Design review of the part built by this model. Coordinates are the model's own, in mm. Face numbers are marked on the shaded views. A direction names the side the tool comes from. Give positions to 0.01 mm unless a question says otherwise; leave off trailing zeros. Write each loop counter-clockwise with the first axis right and the second up, starting at its lowest first coordinate (ties: lowest second). Pieces come first, ordered by that corner, then holes. Notation, with made-up numbers: (35, 72.5) - (81, 72.5) arc R12 ccw to (81, 76.5) - close; hole circle Ø2 at (-1, -24.75). An arc over 180 degrees is marked (long way). Write each question's results on one line, items separated by ' | '. Start each with the question number.
from build123d import *

# Parameters (mm, degrees)
F0_W     = 23
F0_H     = 35
F1_DEPTH = 4.25
F2_W     = 3.5
F2_H     = 35
F3_DEPTH = 17
F4_W     = 6.35
F4_H     = 25
F5_DEPTH = 4.251
F6_R     = 1.15
F7_DEPTH = 3.501


with BuildPart() as f1:
    # F0 (on Front) → F1 (new body)
    with BuildSketch(Plane.XZ):
        with Locations((0.065487, 0)):
            Rectangle(F0_W, F0_H)
    extrude(amount=-F1_DEPTH)

    # F2 (on face) → F3 (join)
    with BuildSketch(Plane.XZ):
        with Locations((-9.684513, 0)):
            Rectangle(F2_W, F2_H)
    extrude(amount=F3_DEPTH)

    # F4 (on face) → F5 (cut, through all)
    with BuildSketch(Plane.XZ):
        with Locations((1.815487, 0)):
            Rectangle(F4_W, F4_H)
    extrude(amount=-F5_DEPTH, mode=Mode.SUBTRACT)

    # F6 (on face) → F7 (cut, through all)
    with BuildSketch(Plane.YZ.offset(-7.934513)):
        with Locations((-13, 12.5)):
            Circle(F6_R)
        with Locations((-6, 12.5)):
            Circle(F6_R)
    extrude(amount=-F7_DEPTH, mode=Mode.SUBTRACT)


solid = f1.part
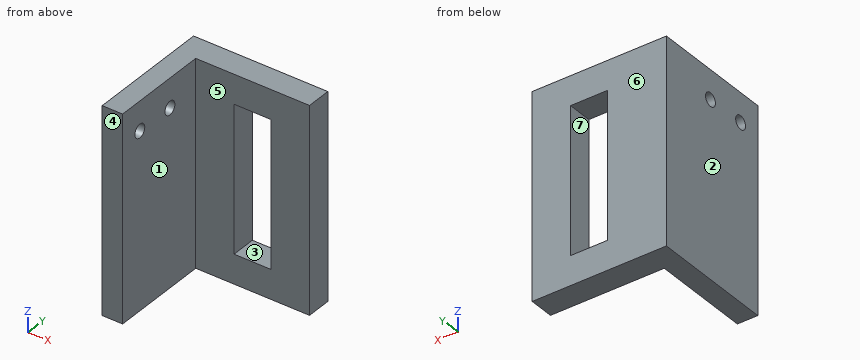
Q1. Add section A-A on z = 8. State the section outline as (x, y) points.
Q2. Add section C-C on y = -6. State the section outline as (x, z) points, plus the area to 3 significant figures.
Q3. Machinability: for the marked faces 5, 6 and 7, which of the approach directions +Z, -Z, +X, -X, +Y, -Y give a long, thin tool a straight path to every point of the face, cutting with its end or side? Answer none if there is none.
Q4. For line 1 along Z through (x, y) = (2.25, 2.25); line 2 along Z through (x, y) = (-9.3, -6); line 3 along X through (y, z) = (1, -0.5), list the stretches that pass through material, from the lowest coordinate up. Write a range as [from, to].
Q5. Add section B-B on x = 4.5. State the section outline as (y, z) points.
Q6. Insertion check: P1, Ø5, axis at y = -3.5, z = -12, coming from the +X side; P2, Ø6, axis at x = 5.5, z = -2.5, coming from the -Y side; P3, Ø1.8, axis at y = -13, z = 12.5, coming from the +X side. Each pin has a flat end and moves straight along its axis. Give the tip position at first contact, or say it passes through.
Q7. Add section D-D on z = -14. State the section outline as (x, y) points.
Q8. The part is to be moulded in two halves that separate along X. For the marked faces 1, 2, 3 and 4, say which applies: +X half, -X half, draft (parallel to the pull), parting line (faces both ways), or undercut.
Result:
1) outline: (-11.43, -17) - (-7.93, -17) - (-7.93, 0) - (-1.36, 0) - (-1.36, 4.25) - (-11.43, 4.25) - close; (4.99, 0) - (11.57, 0) - (11.57, 4.25) - (4.99, 4.25) - close
2) outline: (-11.43, -17.5) - (-7.93, -17.5) - (-7.93, 11.35) - (-11.43, 11.35) - close; (-11.43, 13.65) - (-7.93, 13.65) - (-7.93, 17.5) - (-11.43, 17.5) - close | area: 114 mm²
3) face 5: +Z, -Z, +X, -Y | face 6: +Z, -Z, +X, -X, +Y | face 7: +Y, -Y
4) line 1: z = [-17.5, -12.5], [12.5, 17.5] | line 2: z = [-17.5, 11.35], [13.65, 17.5] | line 3: x = [-11.43, -1.36], [4.99, 11.57]
5) outline: (0, -17.5) - (4.25, -17.5) - (4.25, -12.5) - (0, -12.5) - close; (0, 12.5) - (4.25, 12.5) - (4.25, 17.5) - (0, 17.5) - close
6) P1: stops at x = -7.93 | P2: stops at y = 0 | P3: passes through
7) outline: (-11.43, -17) - (-7.93, -17) - (-7.93, 0) - (11.57, 0) - (11.57, 4.25) - (-11.43, 4.25) - close
8) face 1: +X half | face 2: -X half | face 3: undercut | face 4: draft
